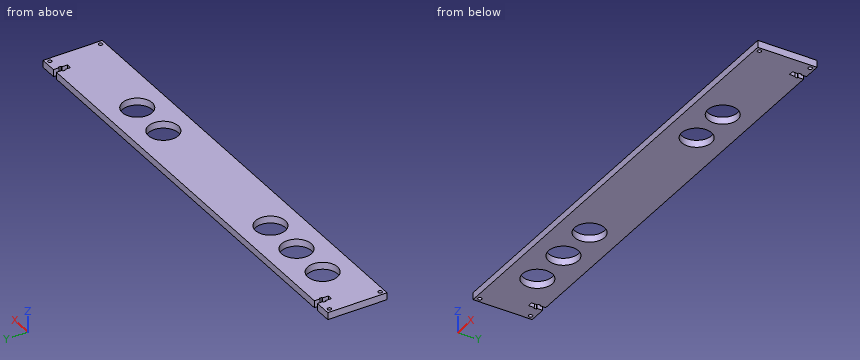
from build123d import *

# Parameters (mm, degrees)
SKETCH1_W                   = 415.925
SKETCH1_H                   = 53.34
BOSS_EXTRUDE1_DEPTH         = 6.35
SKETCH6_R                   = 13.462
CUT_EXTRUDE4_DEPTH          = 502.480799104
F_29_0_136_DIAMETER_HOLE1_D = 3.4544
CUT_EXTRUDE3_DEPTH          = 502.480799104


with BuildPart() as part:
    # Sketch1 → Boss-Extrude1 (new body)
    with BuildSketch(Plane.XY):
        with Locations((-250.890650119, 175.558721987)):
            Rectangle(SKETCH1_W, SKETCH1_H)
    extrude(amount=BOSS_EXTRUDE1_DEPTH)

    # Sketch6 → Cut-Extrude4 (cut, through all)
    with BuildSketch(Plane.XY.offset(6.35)):
        with Locations((-408.053150119, 175.558721987)):
            Circle(SKETCH6_R)
        with Locations((-175.467685368, 175.558721987)):
            Circle(SKETCH6_R)
        with Locations((-369.953150119, 175.558721987)):
            Circle(SKETCH6_R)
        with Locations((-331.853150119, 175.558721987)):
            Circle(SKETCH6_R)
        with Locations((-137.367685368, 175.558721987)):
            Circle(SKETCH6_R)
    extrude(amount=-CUT_EXTRUDE4_DEPTH, mode=Mode.SUBTRACT)

    # #29 (0.136) Diameter Hole1 (through all)
    with Locations(Plane.XY.offset(6.35)):
        with Locations((-455.043150119, 198.418721987), (-455.043150119, 152.698721987), (-46.738150119, 198.418721987), (-46.738150119, 152.698721987)):
            Hole(F_29_0_136_DIAMETER_HOLE1_D / 2)

    # Sketch5 → Cut-Extrude3 (cut, through all)
    with BuildSketch(Plane(origin=(0, 0, 0), x_dir=(-1, 0, 0), z_dir=(0, 0, -1))):
        Polygon((443.587750119, 202.228721987), (439.193550119, 202.228721987), (439.193550119, 197.228096987), (438.215650119, 197.228096987), (438.215650119, 194.688096987), (439.193550119, 194.688096987), (439.193550119, 189.528721987), (443.587750119, 189.528721987), (443.587750119, 194.688096987), (444.565650119, 194.688096987), (444.565650119, 197.228096987), (443.587750119, 197.228096987), align=None)
        Polygon((62.587750119, 202.228721987), (58.193550119, 202.228721987), (58.193550119, 197.228096987), (57.215650119, 197.228096987), (57.215650119, 194.688096987), (58.193550119, 194.688096987), (58.193550119, 189.528721987), (62.587750119, 189.528721987), (62.587750119, 194.688096987), (63.565650119, 194.688096987), (63.565650119, 197.228096987), (62.587750119, 197.228096987), align=None)
    extrude(amount=-CUT_EXTRUDE3_DEPTH, mode=Mode.SUBTRACT)


solid = part.part
Here's how the part is built. I have some questions about the finished solid (model axes, mm). Coordinates: 2 decimals unless noted, no trailing zeros. Order: outer loops, then holes, each group sorted by start corner. A loop starts at its lowest first (then second) coordinate and runs counter-clockwise, first axis right, second up. Notation, with made-up numbers: M 39.25,-12 L 76.25,-12 A20 cw 76.25,8 Z; hole C 75,-35.75 d4. An arc over 180 degrees is marked long. Answer as CSV lines item,"result". Start each with the question number.
1. I want a section at B-B, the plane y = 183. Write out the boundary of the cut face in (x, z), and give its area (3 significant figures).
2. I need wall thicknesses on line 1 (X direction, y = 192.5, z = 2.5); line 2 (X direction, y = 175, z = 1.5); line 3 (X direction, y = 153.5, z = 1.75). Which ranges of each line are inside material? Lowest first, please. Write a range as [from, to].
3. I want a section at A-A, the plane x = -170.5. Write out the boundary of the cut face in (y, z).
4. I want a section at D-D, the plane z = 3.5. Count the separate pieces of the cut face and the enclosed holes in it, and give its area (3 significant figures).
5. I want a section at C-C, the plane x = -405.5. Write out the boundary of the cut face in (y, z), and give its area (3 significant figures).
Recorded:
1,outline,"M -458.85,0 L -419.27,0 L -419.27,6.35 L -458.85,6.35 Z; M -396.83,0 L -381.17,0 L -381.17,6.35 L -396.83,6.35 Z; M -358.73,0 L -343.07,0 L -343.07,6.35 L -358.73,6.35 Z; M -320.63,0 L -186.69,0 L -186.69,6.35 L -320.63,6.35 Z; M -164.25,0 L -148.59,0 L -148.59,6.35 L -164.25,6.35 Z; M -126.15,0 L -42.93,0 L -42.93,6.35 L -126.15,6.35 Z"
1,area,"1,930 mm2"
2,line 1,"x = [-458.85, -443.59], [-439.19, -62.59], [-58.19, -42.93]"
2,line 2,"x = [-458.85, -421.5], [-394.6, -383.4], [-356.5, -345.3], [-318.4, -188.92], [-162.02, -150.82], [-123.92, -42.93]"
2,line 3,"x = [-458.85, -456.57], [-453.51, -48.27], [-45.21, -42.93]"
3,outline,"M 148.89,0 L 163.05,0 L 163.05,6.35 L 148.89,6.35 Z; M 188.07,0 L 202.23,0 L 202.23,6.35 L 188.07,6.35 Z"
4,separate pieces,"1"
4,enclosed holes,"9"
4,area,"19,200 mm2"
5,outline,"M 148.89,0 L 162.34,0 L 162.34,6.35 L 148.89,6.35 Z; M 188.78,0 L 202.23,0 L 202.23,6.35 L 188.78,6.35 Z"
5,area,"171 mm2"
